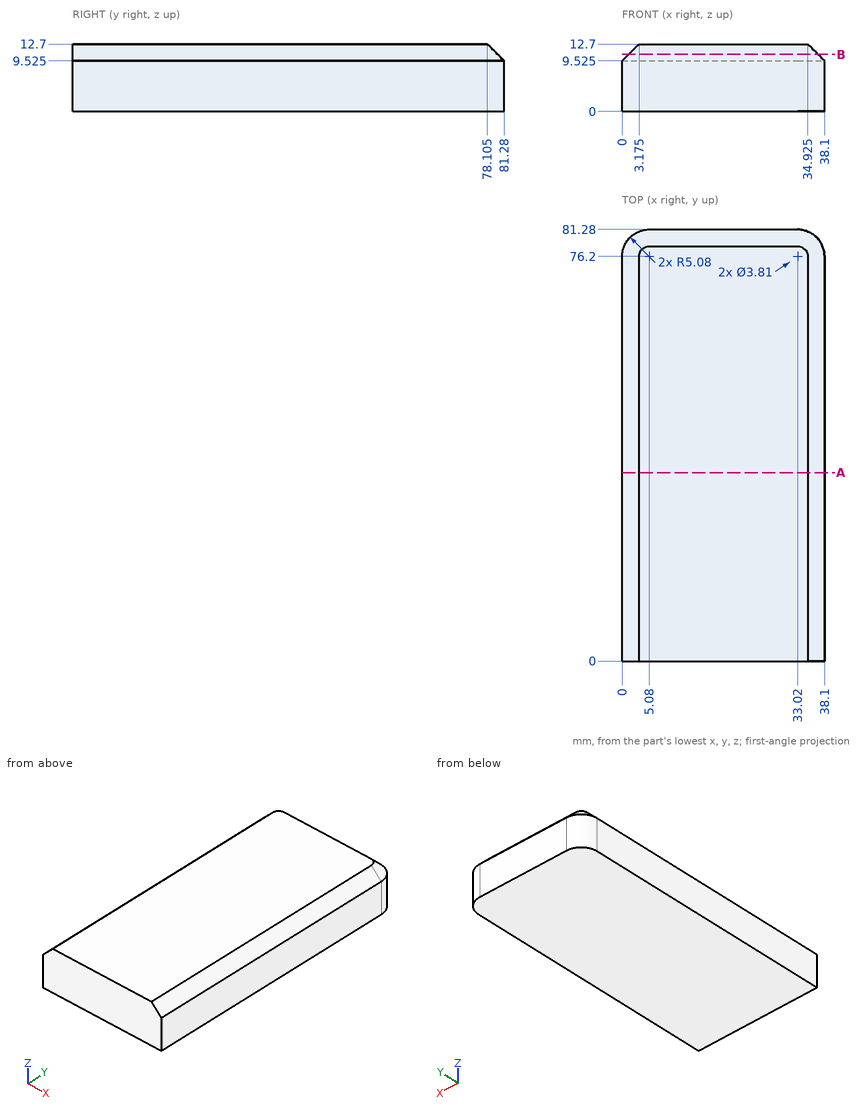
The drawing under review shows one solid part. Ordinate dimensions are in mm from its lowest x, y, z. Give positions to 0.01 mm unless a question says otherwise; leave off trailing zeros. Write each loop counter-clockwise with the first axis right and the second up, starting at its lowest first coordinate (ties: lowest second). Pieces come first, ordered by that corner, then holes. Notation, with made-up numbers: (-37, 59.25) - (6, 59.25) arc R19 cw to (6, 94.25) - close; hole circle Ø5 at (69, 42). An arc over 180 degrees is marked (long way). Answer in a Markdown table with one row per item. Add a question column.
1. We need section B-B on z = 10.75. Write out the cut boundary in (x, y) (3 decimals).
2. We need section A-A on y = 35.5. Write out the cut boundary in (x, z) (3 decimals).
3. Wall thickness on line 1 along Y through (x, z) = (5, 1.5); line 2 along Z through (x, y) = (35, 27) (3 decimals); line 3 along Y through (x, z) = (2, 0.5): over which ranges is each line inside the solid? List them lowest first. Write a range as [from, to].
Ans:
| question | item | result |
|---|---|---|
| 1 | outline | (1.225, 0) - (36.875, 0) - (36.875, 76.2) arc R3.855 ccw to (33.02, 80.055) - (5.08, 80.055) arc R3.855 ccw to (1.225, 76.2) - close |
| 2 | outline | (0, 0) - (38.1, 0) - (38.1, 9.525) - (34.925, 12.7) - (3.175, 12.7) - (0, 9.525) - close |
| 3 | line 1 | y = [0, 81.28] |
| 3 | line 2 | z = [0, 12.625] |
| 3 | line 3 | y = [0, 80.24] |
